Autodesk Inventor part; units mm, degrees
ref_plane "YZ Plane" through (0, 0, 0) normal (1, 0, 0) x (0, 1, 0)
ref_plane "XZ Plane" through (0, 0, 0) normal (0, 1, 0) x (-1, 0, 0)
ref_plane "XY Plane" through (0, 0, 0) normal (0, 0, 1) x (1, 0, 0)
sketch "Skizze1" plane through (0, 0, 0) normal (0, 1, 0) x (-1, 0, 0)
  line L0 (13, 63) -> (-13, 63) construction
  line L1 (0, 63) -> (0, -88) construction
  arc A0 (-35.0888, -80.7018) -> (35.0888, -80.7018) centre (0, 0) ccw construction
  arc A1 (-85.5688, 20.542) -> (-77.3365, -41.9889) centre (0, 0) ccw construction
  arc A2 (77.3365, -41.9889) -> (85.5688, 20.542) centre (0, 0) ccw construction
  line L2 (36.329, -52.1602) -> (44.9364, 46.717) construction
  line L3 (44.9364, 46.717) -> (-44.9364, 46.717) construction
  line L4 (-44.9364, 46.717) -> (-36.329, -52.1602) construction
  line L5 (-36.329, -52.1602) -> (36.329, -52.1602) construction
  line L6 (44.2988, -52.854) -> (52.9063, 46.0232)
  line L7 (44.9364, 54.717) -> (-44.9364, 54.717)
  line L8 (-52.9063, 46.0232) -> (-44.2988, -52.854)
  line L9 (-36.329, -60.1602) -> (36.329, -60.1602)
  arc A3 (36.329, -60.1602) -> (44.2988, -52.854) centre (36.329, -52.1602) ccw
  arc A4 (-44.2988, -52.854) -> (-36.329, -60.1602) centre (-36.329, -52.1602) ccw
  arc A5 (-44.9364, 54.717) -> (-52.9063, 46.0232) centre (-44.9364, 46.717) ccw
  arc A6 (52.9063, 46.0232) -> (44.9364, 54.717) centre (44.9364, 46.717) ccw
  line L10 (43.6628, -60.1602) -> (53.6631, 54.717)
  line L11 (53.6631, 54.717) -> (-53.6631, 54.717)
  line L12 (-53.6631, 54.717) -> (-43.6628, -60.1602)
  line L13 (-43.6628, -60.1602) -> (43.6628, -60.1602)
  arc A7 (-43.6628, -60.1602) -> (43.6628, -60.1602) centre (0, 50.7799) ccw
  arc A8 (53.6631, 54.717) -> (-53.6631, 54.717) centre (0, -114.9743) ccw
  line L14 (0, 63) -> (0, 51)
  line L15 (6, 51) -> (-6, 51)
  line L16 (-6, 51) -> (-6, 63)
  line L17 (-6, 63) -> (6, 63)
  line L18 (6, 63) -> (6, 51)
  line L19 (6, 51) -> (-6, 63) construction
  line L20 (-6, 51) -> (6, 63) construction
  line L21 (0, -68.4432) -> (0, -56.4432)
  line L22 (6, -68.4432) -> (-6, -68.4432)
  line L23 (-6, -68.4432) -> (-6, -56.4432)
  line L24 (-6, -56.4432) -> (6, -56.4432)
  line L25 (6, -56.4432) -> (6, -68.4432)
  line L26 (6, -68.4432) -> (-6, -56.4432) construction
  line L27 (-6, -68.4432) -> (6, -56.4432) construction
  circle A9 centre (0, 0) radius 88
  point P0 (0, 0)
  point P1 (136.7943, -100.6712)
  point P2 (133.0243, -72.1229)
  point P3 (126.2508, -68.622)
  point P4 (131.1382, -105.7457)
  point P5 (170.7312, -118.661)
  point P6 (170.703, -118.661)
  point P7 (165.9867, -123.8079)
  point P8 (170.7158, -118.647)
  point P9 (181.0377, -128.1052)
  point P10 (176.3086, -133.2662)
  point P11 (-44.9364, 54.717)
  point P12 (-44.9364, 54.717)
  point P13 (0, 57)
  point P14 (0, -62.4432)
  point P15 (0, -62.4432)
  point P16 (0, 57)
  point P17 (6, -68.2921)
  point P18 (-6, -68.2921)
  point P19 (-6, 62.8988)
  point P20 (6, 62.8988)
  dimension "d27" = 72.6579
  dimension "d28" = 89.8728
  dimension "d29" = 8
  dimension "d30" = 8
  dimension "d38" = 8
  dimension "d43" = 12
  dimension "d44" = 12
  dimension "d45" = 12
  dimension "d46" = 12
extrude "Extrusion1" add sketch "Skizze1" against normal blind 1.5 contours A3 L9 L25 L24 L23 A4 L8 A5 L7 L16 L15 L18 A6 L6 | L10 L13 A3 | A6 L11 L10 | L13 A7 L25 L9 | L7 L18 A8 L11 | L25 A7 L21 L9 | L9 L21 L24 L25 | L18 L15 L14 L7 | L7 L14 A8 L18 | L21 A7 L23 L9 | L9 L23 L24 L21 | L14 L15 L16 L7 | L7 L16 A8 L14 | L23 A7 L13 L9 | L7 L11 A8 L16 | L13 L12 A4 | A5 L12 L11
hole "Bohrung1" at (36.329, 0, -52.1602) at (44.9364, 0, 46.717) at (0, 0, 0) at (-36.329, 0, -52.1602) at (-44.9364, 0, 46.717) direction (0, -1, 0) diameter 4.2 depth 1.5
hole "Bohrung2" at (0, 0, 57) at (0, 0, -62.4432) direction (0, -1, 0) diameter 3.2 depth 1.5
fillet "Rundung2" radius 8 4 edges at (53.6631, -0.75, 54.717) (43.6628, -0.75, -60.1602) (-43.6628, -0.75, -60.1602) (-53.6631, -0.75, 54.717)
properties part number "Spiegelhalterung"
CAD build for the part. Positions are in the model's coordinates, mm. Give positions to 0.01 mm unless a question says otherwise; leave off trailing zeros. Order: outer loops, then holes, each group sorted by start corner. A loop starts at its lowest first (then second) coordinate and runs counter-clockwise, first axis right, second up. Notation, with made-up numbers: M -16,9 L 12,9 A22 ccw 12,44 Z; hole C 4,61.25 d11. An arc over 180 degrees is marked long. Put each result on its own line as item: value. Start each with the question number.
(1) Saw through at A-A, the plane x = 0. Write the cut outline in (y, z).
(2) Saw through at D-D, the plane z = 21. Write the cut outline in (x, y), then the cut area to 3 significant figures.
(3) Flat gauge pin, fed straight in: pin 1 Ø3.5 at (x, z) = (36.33, -52.16) entering from -Y. Where does the tip first touch, or does it go through?
(4) Mould opens along Z. For faces 1 (the cylindrical face through (-0.7, -0.7, 63)), 2 (the cylindrical face through (0.55, -0.74, -68.44)), 3 (the cylindrical face through (46.986, -0.76, 46.262)) say: +Z half, -Z half, draft (parallel to the pull), parting line (faces both ways), or undercut.
(5) Saw through at B-B, the plane y = -0.7. Write the cut outline in (x, z).
(6) Drill centre lines: line 1 along Z through (x, y) = (0, -0.5); line 2 along X through (y, z) = (-0.7, 45); line 3 along X through (y, z) = (-0.6, -53.5). Where is each one in solid material? Low to high.
(7) Saw through at C-C, the plane z = 0. Write the cut outline in (x, y).
Check result:
1. outline: M -1.5,-68.44 L 0,-68.44 L 0,-64.04 L -1.5,-64.04 Z; M -1.5,-60.84 L 0,-60.84 L 0,-2.1 L -1.5,-2.1 Z; M -1.5,2.1 L 0,2.1 L 0,55.4 L -1.5,55.4 Z; M -1.5,58.6 L 0,58.6 L 0,63 L -1.5,63 Z
2. outline: M -50.73,-1.5 L 50.73,-1.5 L 50.73,0 L -50.73,0 Z
2. area: 152 mm2
3. pin 1: passes through
4. face 1: +Z half
4. face 2: -Z half
4. face 3: undercut
5. outline: M -53.1,48.21 L -52.91,46.02 L -44.3,-52.85 L -44.1,-55.1 A8 ccw -38.73,-61.98 A119.22 ccw 38.73,-61.98 A8 ccw 44.1,-55.1 L 44.3,-52.85 L 52.91,46.02 L 53.1,48.21 A8 ccw 47.25,56.61 A177.97 ccw -47.25,56.61 A8 ccw Z; hole C -44.94,46.72 d4.2; hole C -36.33,-52.16 d4.2; hole C 0,0 d4.2; hole C 0,-62.44 d3.2; hole C 0,57 d3.2; hole C 36.33,-52.16 d4.2; hole C 44.94,46.72 d4.2
6. line 1: z = -68.44 to -64.04, -60.84 to -2.1, 2.1 to 55.4, 58.6 to 63
6. line 2: x = -52.82 to -46.15, -43.73 to 43.73, 46.15 to 52.82
6. line 3: x = -44.24 to -37.95, -34.71 to 34.71, 37.95 to 44.24
7. outline: M -48.9,-1.5 L -2.1,-1.5 L -2.1,0 L -48.9,0 Z; M 2.1,-1.5 L 48.9,-1.5 L 48.9,0 L 2.1,0 Z
